Geometry: final body of the model. Coordinates: model frame, mm. Face numbers are marked on the shaded views. A direction names the side the tool comes from. Give positions to 0.01 mm unless a question says otherwise; leave off trailing zeros. Write each loop counter-clockwise with the first axis right and the second up, starting at its lowest first coordinate (ties: lowest second). Pieces come first, ordered by that corner, then holes. Notation, with made-up numbers: M 18.25,43 L 39.25,43 A26 ccw 39.25,58 Z; hole C 26,48 d7. An arc over 180 degrees is marked long. Use one line per item in the form item = value. Start each with the question number.
Item 1: Pull-direction query (Y, two-part tool) for the marked faces 3, 4 and 5; classes: released by +Y, released by -Y, zero draft, split by the parting line, or undercut.
Item 2: Section query D-D on z = 12.75. Return loops of the section in (x, y), then the cut area to 3 significant figures.
Item 3: Contact query for a flat-ended pin moving along its axis: P1, Ø2, axis at x = -1.5, y = 2, coming from the +Z side. Output: stop coordinate, or through.
Item 4: Access query for the marked faces 1 and 2. Directions: +Z, -Z, +X, -X, +Y, -Y. A direction counts if a zero-diameter tool reaches every point of the face in a straight line with its end or side. Return the directions, or none.
Item 5: Section query B-B on x = 0. Return loops of the section in (y, z).
Item 6: Section query A-A on z = 2.75. Return loops of the section in (x, y).
Item 7: Material intervals for line 1 along Y through (x, z) = (0, 3.25); line 2 along Z through (x, y) = (2.25, -0.3); line 3 along Z through (x, y) = (0.35, 0.25), sorted ascending. Write a range as from..to.
Item 8: Section query C-C on y = 0.85. Return loops of the section in (x, z).
from build123d import *

# Parameters (mm, degrees)
BODY_DEPTH                      = 10
SKIZZE2_R                       = 1.25
THREAD_DEPTH                    = 4.75
SKIZZE3_R                       = 1.25
SCHNITT_LINEAR_AUSTRAGEN1_DEPTH = 6.4


with BuildPart() as part:
    # Skizze1 → Body (new body)
    with BuildSketch(Plane.XY):
        Polygon((2.655811238, 0), (1.327905619, 2.3), (-1.327905619, 2.3), (-2.655811238, 0), (-1.327905619, -2.3), (1.327905619, -2.3), align=None)
    extrude(amount=BODY_DEPTH)

    # Skizze2 → Thread (add)
    with BuildSketch(Plane.XY.offset(10)):
        Circle(SKIZZE2_R)
    extrude(amount=THREAD_DEPTH)

    # Skizze3 → Schnitt-Linear austragen1 (cut)
    with BuildSketch(Plane(origin=(0, 0, 0), x_dir=(-1, 0, 0), z_dir=(0, 0, -1))):
        with Locations(Location((0, 0, 0), (0, 0, 180))):
            Circle(SKIZZE3_R)
    extrude(amount=-SCHNITT_LINEAR_AUSTRAGEN1_DEPTH, mode=Mode.SUBTRACT)


solid = part.part
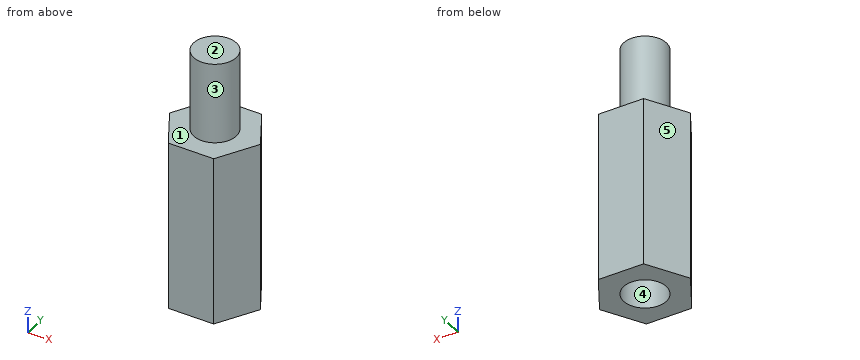
Answer sheet:
q1.face_3 = split by the parting line
q1.face_4 = undercut
q1.face_5 = released by +Y
q2.outline = C 0,0 d2.5
q2.area = 4.91 mm2
q3.P1 = 10
q4.face_1 = +Z
q4.face_2 = +Z, +X, -X, +Y, -Y
q5.outline = M -2.3,0 L -1.25,0 L -1.25,6.4 L 1.25,6.4 L 1.25,0 L 2.3,0 L 2.3,10 L 1.25,10 L 1.25,14.75 L -1.25,14.75 L -1.25,10 L -2.3,10 Z
q6.outline = M -2.66,0 L -1.33,-2.3 L 1.33,-2.3 L 2.66,0 L 1.33,2.3 L -1.33,2.3 Z; hole C 0,0 d2.5
q7.line_1 = -2.3..-1.25, 1.25..2.3
q7.line_2 = 0..10
q7.line_3 = 6.4..14.75
q8.outline = M -2.17,0 L -0.92,0 L -0.92,6.4 L 0.92,6.4 L 0.92,0 L 2.17,0 L 2.17,10 L 0.92,10 L 0.92,14.75 L -0.92,14.75 L -0.92,10 L -2.17,10 Z
